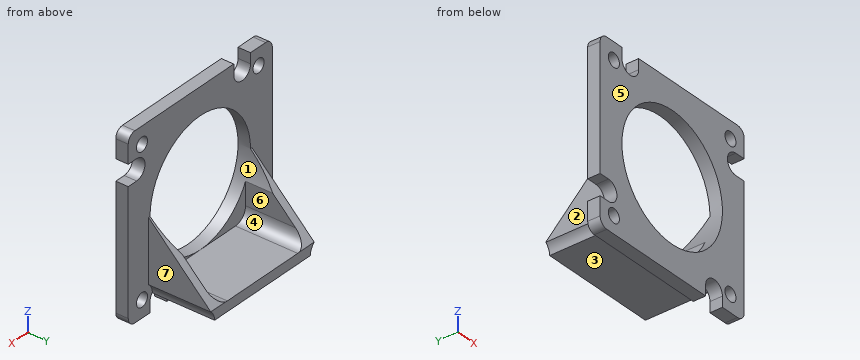
Autodesk Inventor part; units mm, degrees
ref_plane "YZ Plane" through (0, 0, 0) normal (1, 0, 0) x (0, 1, 0)
ref_plane "XZ Plane" through (0, 0, 0) normal (0, 1, 0) x (-1, 0, 0)
ref_plane "XY Plane" through (0, 0, 0) normal (0, 0, 1) x (1, 0, 0)
sketch "Эскиз1" plane through (0, 0, 0) normal (0, 1, 0) x (-1, 0, 0)
  arc A0 (82, -4) -> (78, 0) centre (78, -4) ccw
  line L0 (82, -63) -> (82, -4)
  line L1 (-4, -23) -> (-4, -82)
  line L2 (1, -23) -> (-4, -23)
  arc A1 (1, -23) -> (6, -18) centre (1, -18) ccw
  arc A2 (6, -18) -> (1, -13) centre (1, -18) ccw
  circle A3 centre (39, -43) radius 30
  line L3 (-4, -13) -> (1, -13)
  line L4 (-4, -4) -> (-4, -13)
  arc A4 (0, 0) -> (-4, -4) centre (0, -4) ccw
  line L5 (59, 0) -> (0, 0)
  line L6 (59, -5) -> (59, 0)
  line L7 (78, 0) -> (69, 0)
  arc A5 (59, -5) -> (69, -5) centre (64, -5) ccw
  line L8 (69, 0) -> (69, -5)
  arc A6 (77.1, -8.2) -> (70.5, -8.2) centre (73.8, -8.2) ccw
  circle A7 centre (73.8, -8.2) radius 3.3
  circle A8 centre (4.2, -8.2) radius 3.3
  circle A9 centre (73.8, -77.8) radius 3.3
  circle A10 centre (4.2, -77.8) radius 3.3
  arc A11 (19, -81) -> (9, -81) centre (14, -81) ccw
  line L9 (19, -81) -> (19, -86)
  line L10 (9, -86) -> (9, -81)
  line L11 (0, -86) -> (9, -86)
  arc A12 (-4, -82) -> (0, -86) centre (0, -82) ccw
  line L12 (19, -86) -> (78, -86)
  arc A13 (78, -86) -> (82, -82) centre (78, -82) ccw
  line L13 (82, -82) -> (82, -73)
  line L14 (82, -73) -> (77, -73)
  arc A14 (77, -63) -> (77, -73) centre (77, -68) ccw
  line L15 (77, -63) -> (82, -63)
  point P0 (0, 0)
extrude "Выдавливание1" add sketch "Эскиз1" along normal blind 6
sketch "Эскиз2" plane through (0, 6, 0) normal (0, 1, 0) x (1, 0, 0)
  line L0 (4, 23) -> (4, 82)
  line L1 (-82, 85.8) -> (4, 85.8)
  line L2 (4, 85.8) -> (4, 77.8)
  line L3 (4, 77.8) -> (-82, 77.8)
  line L4 (-82, 77.8) -> (-82, 85.8)
  circle A0 centre (-73.8, 77.8) radius 3.3
  circle A1 centre (-4.2, 77.8) radius 3.3
  circle A2 centre (-4.2, 77.8) radius 6.2032
  circle A3 centre (-73.8, 77.8) radius 6.2032
  line L5 (-82, 73) -> (-77, 73)
  line L6 (-82, 73) -> (4, 73)
  line L7 (4, 73) -> (4, 77.8)
  line L8 (4, 77.8) -> (-82, 77.8)
  line L9 (-82, 77.8) -> (-82, 73)
  line L10 (-8.1294, 73) -> (-12, 73)
  line L11 (-12, 73) -> (-12, 42.9076)
  line L12 (-12, 42.9076) -> (-8.1294, 42.9076)
  line L13 (-8.1294, 42.9076) -> (-8.1294, 73)
  line L14 (-69.8706, 73) -> (-66.037, 73)
  line L15 (-66.037, 73) -> (-66.037, 42.9076)
  line L16 (-66.037, 42.9076) -> (-69.8706, 42.9076)
  line L17 (-69.8706, 42.9076) -> (-69.8706, 73)
  circle A4 centre (-39, 43) radius 30
  point P0 (0, 0)
  point P1 (-80.0032, 77.8)
  point P2 (-67.5968, 77.8)
  point P3 (-10.4032, 77.8)
  point P4 (2.0032, 77.8)
  point P5 (-12, 56.0767)
  point P6 (-9.0001, 42.9076)
  point P7 (-68.9999, 42.9076)
  point P8 (-66.037, 56)
  dimension "d4" = 4.8
  dimension "d5" = 8
extrude "Выдавливание3" add sketch "Эскиз2" along normal blind 30 contours L6 A3 L3 A2 | L13 L12 A4 L11 L6 | L6 L15 A4 L16 L17
chamfer "Фаска1" distance 30 angle 45 2 edges at (-69.4352, 36, -42.9076) (-8.5648, 36, -42.9076)
fillet "Сопряжение1" radius 6 2 edges at (-66.037, 21, -73) (-12, 21, -73)
properties part number "MotorCrepper2"
Geometry check sheet. Reference: the model listing, model coordinates, mm. Face numbers are marked on the shaded views. A direction names the side the tool comes from. Give positions to 0.01 mm unless a question says otherwise; leave off trailing zeros. Order: outer loops, then holes, each group sorted by start corner. A loop starts at its lowest first (then second) coordinate and runs counter-clockwise, first axis right, second up.
1. Section check A-A, the plane x = -57. Enter the section's corners in (y, z), and give its area (3 significant figures).
2. Access from +Z, -Z, +X, -X, +Y, -Y to the whole of each face (thin tool, end or side, straight path). Record for the marked faces 1, 2, 3 and 4.
3. Section check D-D, the plane z = -70. Enter the section's corners in (x, y), and give its area (3 significant figures).
4. Gauge pin test, flat ends, axial feed: pin 1 Ø6 at (x, y) = (-51.5, 15.5) entering from -Z; pin 2 Ø1.5 at (x, y) = (-61, 28.5) entering from +Z; pin 3 Ø15 at (x, y) = (-31.5, 17) entering from +Z; pin 4 Ø5 at (x, z) = (-50.5, -66.5) entering from +Y. Record the tip position at first contact, or that the pin passes through.
5. Section check C-C, the plane y = 4. Give the number of separate pieces and of enclosed holes in the cut face, and give its area (3 significant figures).
6. Thickness scan on L1, parallel to Z at x = -73.8, y = 4.6; L2, parallel to Z at x = -37, y = 10; L3, parallel to X at y = 5, z = -43. Record the ranges inside material, lowest first.
7. Section check B-B, the plane z = -8.2. Enter the section's corners in (x, y).
8. Release check for a two-part mould opening along X. For the marked faces 5, 6 and 7 record: pulls with the +X half, pulls with the -X half, needs draft (parallel to the pull), parting line crosses it, or undercut.
Values follow:
1. outline: (0, -86) - (6, -86) - (6, -77.8) - (36, -77.8) - (36, -73) - (6, -73) - (6, -67) - (0, -67) - close; (0, -19) - (6, -19) - (6, 0) - (0, 0) - close
1. area: 372 mm2
2. face 1: +Y, -Y
2. face 2: +Z, -Z, -X, +Y
2. face 3: -Z, +X, -X, +Y
2. face 4: +Z, +Y
3. outline: (-72.42, 0) - (-52.08, 0) - (-52.08, 6) - (-65.23, 6) - (-65.23, 33.09) - (-69.87, 33.09) - (-69.87, 6) - (-72.42, 6) - close; (-25.92, 0) - (4, 0) - (4, 6) - (-8.13, 6) - (-8.13, 33.09) - (-12.8, 33.09) - (-12.8, 6) - (-25.92, 6) - close
3. area: 554 mm2
4. pin 1: stops at z = -77.8
4. pin 2: stops at z = -72.75
4. pin 3: stops at z = -73
4. pin 4: passes through
5. separate pieces: 1
5. enclosed holes: 5
5. area: 4,060 mm2
6. L1: z = -86 to -81.1, -74.5 to -71.84, -64.16 to -11.5, -4.9 to 0
6. L2: z = -77.8 to -73
6. L3: x = -82 to -69, -9 to 4
7. outline: (-82, 0) - (-77.1, 0) - (-77.1, 6) - (-82, 6) - close; (-70.5, 0) - (-67.84, 0) - (-67.84, 6) - (-70.5, 6) - close; (-60.16, 0) - (-7.5, 0) - (-7.5, 6) - (-60.16, 6) - close; (-0.9, 0) - (4, 0) - (4, 6) - (-0.9, 6) - close
8. face 5: needs draft
8. face 6: undercut
8. face 7: pulls with the +X half
